```python
from build123d import *

# Parameters (mm, degrees)
F0_W      = 80
F0_H      = 63
F0_W_2    = 78
F0_H_2    = 61
F1_DEPTH  = 13
F3_DEPTH  = 63
F4_T      = -2.4
F5_DEPTH  = 2
F6_DEPTH  = 1.6
F7_W      = 7.2
F7_H      = 6.2
F8_DEPTH  = 2
F9_W      = 12
F9_H      = 12
F10_DEPTH = 1.4
F9_H_2    = 1.5
F11_DEPTH = 3
F12_W     = 12
F12_H     = 11.6
F13_DEPTH = 1.6
F14_W     = 7.2
F14_H     = 4.8
F15_DEPTH = 3
F16_DEPTH = 1
F2_W      = 6
F2_H      = 1
F17_DEPTH = 1
F18_DEPTH = 1


with BuildPart() as f1:
    # F0 (on Top) → F1 (new body)
    with BuildSketch(Plane.XY):
        Rectangle(F0_W, F0_H)
        Rectangle(F0_W_2, F0_H_2, mode=Mode.SUBTRACT)
        Rectangle(F0_W_2, F0_H_2)
    extrude(amount=F1_DEPTH)

    # F2 (on face) → F3 (cut)
    with BuildSketch(Plane.XZ.offset(31.5)):
        Polygon((-39.5, 13), (-40, 13), (-40, 0), align=None)
        Polygon((39.5, 13), (40, 0), (40, 13), align=None)
    extrude(amount=-F3_DEPTH, mode=Mode.SUBTRACT)

    # F4
    f4_openings = [f1.faces().sort_by_distance(p)[0] for p in [
        (0, 0, 0),
    ]]
    offset(amount=F4_T, openings=f4_openings)

    # F0 (on Top) → F5 (cut)
    with BuildSketch(Plane.XY):
        Rectangle(F0_W_2, F0_H_2)
    extrude(amount=F5_DEPTH, mode=Mode.SUBTRACT)

    # F2 (on face) → F6 (cut)
    with BuildSketch(Plane.XZ.offset(31.5)):
        Polygon((18, 2.6), (18, 0), (30, 0), (30, 13), (18, 13), (18, 3.6), align=None)
    extrude(amount=-F6_DEPTH, mode=Mode.SUBTRACT)

    # F7 (on face) → F8 (cut)
    with BuildSketch(Plane.XZ.offset(29.9)):
        with Locations((24, 7.5)):
            Rectangle(F7_W, F7_H)
    extrude(amount=-F8_DEPTH, mode=Mode.SUBTRACT)

    # F9 (on face) → F10 (cut)
    with BuildSketch(Plane.XY.offset(13)):
        with Locations((24, 25.5)):
            Rectangle(F9_W, F9_H)
        Polygon((18, -20.5), (18, -29.9), (30, -29.9), (30, -19.5), (18, -19.5), align=None)
    extrude(amount=-F10_DEPTH, mode=Mode.SUBTRACT)

    # F9 (on face) → F11 (cut)
    with BuildSketch(Plane.XY.offset(13)):
        with Locations((24, -17.25)):
            Rectangle(F9_W, F9_H_2)
        with Locations((24, -14.25)):
            Rectangle(F9_W, F9_H_2)
        with Locations((24, -11.25)):
            Rectangle(F9_W, F9_H_2)
        with Locations((24, -8.25)):
            Rectangle(F9_W, F9_H_2)
        with Locations((24, -5.25)):
            Rectangle(F9_W, F9_H_2)
        with Locations((24, 0.75)):
            Rectangle(F9_W, F9_H_2)
        with Locations((24, -2.25)):
            Rectangle(F9_W, F9_H_2)
        with Locations((24, 3.75)):
            Rectangle(F9_W, F9_H_2)
        with Locations((24, 6.75)):
            Rectangle(F9_W, F9_H_2)
        with Locations((24, 9.75)):
            Rectangle(F9_W, F9_H_2)
        with Locations((24, 12.75)):
            Rectangle(F9_W, F9_H_2)
        with Locations((24, 15.75)):
            Rectangle(F9_W, F9_H_2)
        with Locations((24, 18.75)):
            Rectangle(F9_W, F9_H_2)
    extrude(amount=-F11_DEPTH, mode=Mode.SUBTRACT)

    # F12 (on face) → F13 (cut)
    with BuildSketch(Plane(origin=(0, 31.5, 0), x_dir=(-1, 0, 0), z_dir=(0, 1, 0))):
        with Locations((-24, 5.8)):
            Rectangle(F12_W, F12_H)
    extrude(amount=-F13_DEPTH, mode=Mode.SUBTRACT)

    # F14 (on face) → F15 (cut)
    with BuildSketch(Plane(origin=(0, 29.9, 0), x_dir=(-1, 0, 0), z_dir=(0, 1, 0))):
        with Locations((-24, 6.8)):
            Rectangle(F14_W, F14_H)
    extrude(amount=-F15_DEPTH, mode=Mode.SUBTRACT)

    # F9 (on face) → F16 (cut)
    with BuildSketch(Plane.XY.offset(13)):
        Polygon((-29, -20.5), (18, -20.5), (18, -19.5), (-30, -19.5), (-30, -31.5), (-29, -31.5), align=None)
    extrude(amount=-F16_DEPTH, mode=Mode.SUBTRACT)

    # F2 (on face) → F17 (join)
    with BuildSketch(Plane.XZ.offset(31.5)):
        with Locations((-5.5, 4.1)):
            Rectangle(F2_W, F2_H)
    extrude(amount=F17_DEPTH)

    # F2 (on face) → F18 (cut)
    with BuildSketch(Plane.XZ.offset(31.5)):
        Polygon((-29, 13), (-30, 13), (-30, 2.6), (-29, 2.6), (-29, 3.6), align=None)
        Polygon((-29, 2.6), (18, 2.6), (18, 3.6), (-2.5, 3.6), (-8.5, 3.6), (-29, 3.6), align=None)
    extrude(amount=-F18_DEPTH, mode=Mode.SUBTRACT)


solid = f1.part
```
Geometry: final body of the model. Coordinates: model frame, mm. A direction names the side the tool comes from. Round coordinates to 2 decimals unless told otherwise and drop trailing zeros. Write each loop counter-clockwise with the first axis right and the second up, starting at its lowest first coordinate (ties: lowest second). Pieces come first, ordered by that corner, then holes.
Item 1: Section query D-D (x = 32). Return loops of the section in (y, z), plus the area to 3 significant figures.
Item 2: Material intervals for L1, parallel to Y at x = -29.5, z = 7; L2, parallel to Y at x = -26, z = 2.5; L3, parallel to Z at x = 8, y = -25.5, sorted ascending.
Item 3: Mould query, pull axis Y, two halves, no side actions, for faces 5 (the face through (24, -7.5, 12)), 6 (the face through (30, -30.4, 9.4)), 7 (the face through (-11, 31.5, 6)), 8 (the face through (24, -12, 12)). Classes: +Y half, -Y half, draft (parallel to the pull), parting line (faces both ways), or undercut.
Item 4: Section query A-A (x = 3.5). Return loops of the section in (y, z), plus the area to 3 significant figures.
Item 5: Section query B-B (z = 6.25). Return loops of the section in (x, y), plus the area to 3 significant figures.
Item 6: Set-up query: faces 1 (the face through (-29, -28.5, 12.2)), 2 (the face through (24, 1.5, 12)), 3 (the face through (-5, -31, 3.6)), 4 (the face through (37.354, -0.407, 6.36)). Return all of +Z, -Z, +X, -X, +Y, -Y with unobstructed straight access to the full face (end or side cutting, diameter ignored); none if empty.
Item 7: Pin query (flat end, axial travel): P1, Ø6, axis at y = 5, z = 11, coming from the -X side; P2, Ø5, axis at x = 19, y = 8, coming from the -Z side; P3, Ø11.5, axis at x = 23.5, y = -23, coming from the +Z side; P4, Ø1.2, axis at y = -14.5, z = 12, coming from the -X side. Return the tip coordinate at first contact, or that it passes through.
Item 8: Section query C-C (y = -25). Return loops of the section in (x, z), plus the area to 3 significant figures.
Completed:
1. outline: (-31.5, 0) - (-30.5, 0) - (-30.5, 2) - (-29.1, 2) - (-29.1, 10.6) - (29.1, 10.6) - (29.1, 2) - (30.5, 2) - (30.5, 0) - (31.5, 0) - (31.5, 13) - (-31.5, 13) - close
1. area: 196 mm2
2. L1: y = -30.5 to -29.1, 29.1 to 31.5
2. L2: y = -31.5 to -29.1, 29.1 to 31.5
2. L3: z = 10.6 to 13
3. face 5: undercut
3. face 6: draft
3. face 7: +Y half
3. face 8: undercut
4. outline: (-31.5, 0) - (-30.5, 0) - (-30.5, 2) - (-29.1, 2) - (-29.1, 10.6) - (29.1, 10.6) - (29.1, 2) - (30.5, 2) - (30.5, 0) - (31.5, 0) - (31.5, 13) - (-19.5, 13) - (-19.5, 12) - (-20.5, 12) - (-20.5, 13) - (-31.5, 13) - (-31.5, 3.6) - (-30.5, 3.6) - (-30.5, 2.6) - (-31.5, 2.6) - close
4. area: 194 mm2
5. outline: (-39.76, -31.5) - (-30, -31.5) - (-30, -30.5) - (-29, -30.5) - (-29, -31.5) - (18, -31.5) - (18, -29.9) - (20.4, -29.9) - (20.4, -29.1) - (-37.36, -29.1) - (-37.36, 29.1) - (20.4, 29.1) - (20.4, 29.9) - (18, 29.9) - (18, 31.5) - (-39.76, 31.5) - close; (27.6, -29.9) - (30, -29.9) - (30, -31.5) - (39.76, -31.5) - (39.76, 31.5) - (30, 31.5) - (30, 29.9) - (27.6, 29.9) - (27.6, 29.1) - (37.36, 29.1) - (37.36, -29.1) - (27.6, -29.1) - close
5. area: 610 mm2
6. face 1: +Z, -Y
6. face 2: +Z, -Z
6. face 3: -Y
6. face 4: -Z
7. P1: stops at x = -39.69
7. P2: stops at z = 10.6
7. P3: stops at z = 13
7. P4: stops at x = -39.56
8. outline: (-40, 0) - (-39, 0) - (-39, 2) - (-37.52, 2) - (-37.19, 10.6) - (37.19, 10.6) - (37.52, 2) - (39, 2) - (39, 0) - (40, 0) - (39.5, 13) - (30, 13) - (30, 11.6) - (18, 11.6) - (18, 13) - (-29, 13) - (-29, 12) - (-30, 12) - (-30, 13) - (-39.5, 13) - close
8. area: 217 mm2
